Can you work these out from the model? Positions are in its coordinate system, mm. A direction names the side the tool comes from. Round coordinates to 2 decimals unless told otherwise and drop trailing zeros. Write each loop counter-clockwise with the first axis right and the second up, starting at its lowest first coordinate (ties: lowest second). Pieces come first, ordered by that corner, then holes. Notation, with made-up numbers: (30.5, 32.25) -> (46.5, 32.25) arc R19 ccw to (46.5, 64.25) -> close; hole circle Ø2 at (-4, 43.25). An arc over 180 degrees is marked (long way). Use CSV: the item, a comma, the result in double quotes.
```python
from build123d import *

# Parameters (mm, degrees)
SKETCH_W   = 123.6
SKETCH_H   = 200
SKETCH_W_2 = 119.6
SKETCH_H_2 = 196
PAD_DEPTH  = 700


with BuildPart() as part:
    # Sketch → Pad (new body)
    with BuildSketch(Plane.YZ):
        with Locations((61.8, -100)):
            Rectangle(SKETCH_W, SKETCH_H)
        with Locations((61.8, -100)):
            Rectangle(SKETCH_W_2, SKETCH_H_2, mode=Mode.SUBTRACT)
    extrude(amount=PAD_DEPTH)


solid = part.part
```
Q1. Suppose I cut it at B-B (z = -187). Write out the boundary of the cut face in (x, y).
Resolved:
outline,"(0, 0) -> (700, 0) -> (700, 2) -> (0, 2) -> close; (0, 121.6) -> (700, 121.6) -> (700, 123.6) -> (0, 123.6) -> close"
Q2. Suppose I cut it at C-C (x = 511.5). Write out the boundary of the cut face in (y, z), and give its area (3 significant figures).
Resolved:
outline,"(0, -200) -> (123.6, -200) -> (123.6, 0) -> (0, 0) -> close; hole (2, -198) -> (121.6, -198) -> (121.6, -2) -> (2, -2) -> close"
area,"1,280 mm^2"
Q3. On a 3-axis mill with a long thin cutter (end or side, diameter ignored), from which of +Z, -Z, +X, -X, +Y, -Y can I reach the whole of each face in a straight line? I mean faces 4 (the face through (345, 2, -101)), 5 (the face through (345, 0, -101)). Say none if no direction works.
Resolved:
face 4,"+X, -X"
face 5,"+Z, -Z, +X, -X, -Y"
Q4. If we mould it in two halves opening along Z, with no side actions, what happens to faces 1 (the face through (345, 121.6, -101)), 2 (the face through (345, 61, -200)), 3 (the face through (345, 123.6, -101))? For each: released by +Z, released by -Z, zero draft, split by the parting line, or undercut.
Resolved:
face 1,"undercut"
face 2,"released by -Z"
face 3,"zero draft"
Q5. Please list where these lines run through material, in increasing order: probe 1 along Z at (x, y) = (61.5, 33.5); probe 2 along Y at (x, z) = (521.5, -57).
Resolved:
probe 1,"z = -200 to -198, -2 to 0"
probe 2,"y = 0 to 2, 121.6 to 123.6"
Q6. Suppose I cut it at A-A (y = 84). Write out the boundary of the cut face in (x, z).
Resolved:
outline,"(0, -200) -> (700, -200) -> (700, -198) -> (0, -198) -> close; (0, -2) -> (700, -2) -> (700, 0) -> (0, 0) -> close"
